```python
from build123d import *

# Parameters (mm, degrees)
SKETCH1_R                = 10
BOSS_EXTRUDE1_DEPTH      = 30
BOSS_EXTRUDE2_DEPTH      = 100
BOSS_EXTRUDE2_DEPTH_BACK = 30
SKETCH2_W                = 120
SKETCH2_H                = 25
SKETCH3_R                = 5
CUT_EXTRUDE1_DEPTH       = 70


with BuildPart() as part:
    # Sketch1 → Boss-Extrude1 (new body)
    with BuildSketch(Plane(origin=(0, 0, 0), x_dir=(0, 1, 0), z_dir=(0, 0, 1))):
        with BuildLine():
            Line((0, 60), (400, 60))
            Line((400, 60), (460, 60))
            Line((460, 60), (460, -60))
            Line((460, -60), (400, -60))
            Line((400, -60), (0, -60))
            ThreePointArc((0, -60), (-60, 0), (0, 60))
        make_face()
        with Locations(Location((0, 0, 0), (0, 0, 270))):
            Circle(SKETCH1_R, mode=Mode.SUBTRACT)
    extrude(amount=BOSS_EXTRUDE1_DEPTH)

    # Sketch2 → Boss-Extrude2 (add, two sides: drawn at the far end of the back side and taken through both)
    with BuildSketch(Plane.XY.offset(30).offset(-BOSS_EXTRUDE2_DEPTH_BACK)):
        with Locations((0, 472.5)):
            Rectangle(SKETCH2_W, SKETCH2_H)
    extrude(amount=BOSS_EXTRUDE2_DEPTH + BOSS_EXTRUDE2_DEPTH_BACK)

    # Sketch3 → Cut-Extrude1 (cut)
    with BuildSketch(Plane.XZ.offset(-460)):
        with Locations(Location((32, 77, 0), (0, 0, 270))):
            Circle(SKETCH3_R)
    extrude(amount=-CUT_EXTRUDE1_DEPTH, mode=Mode.SUBTRACT)


solid = part.part
```
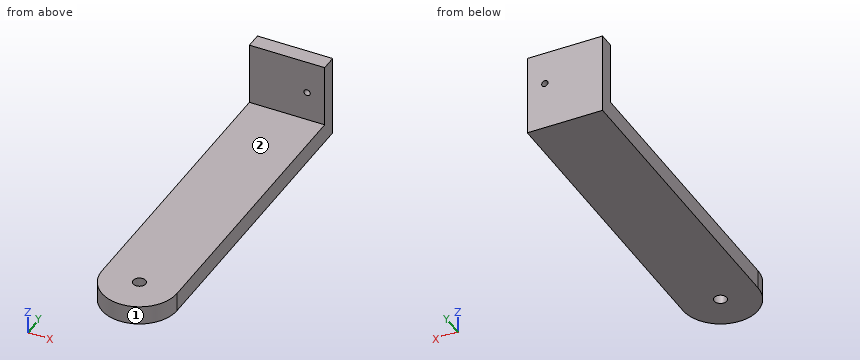
Check sheet for the modelled part. Datum: model origin and axes. Units: mm. Face numbers are marked on the shaded views. A direction names the side the tool comes from. Round coordinates to 2 decimals unless told otherwise and drop trailing zeros. Order: outer loops, then holes, each group sorted by start corner. A loop starts at its lowest first (then second) coordinate and runs counter-clockwise, first axis right, second up.
1) Tool access check on the marked faces 1 and 2. Record the directions out of +Z, -Z, +X, -X, +Y, -Y that give a thin tool (end or side, any length) a straight path to the whole face; none if there is none.
2) Section check C-C (x = 48). Record the boundary of the cut face in (y, z), and give its area (3 significant figures).
3) Section check A-A (z = 77). Record the boundary of the cut face in (x, y).
4) Go/stop test with flat-tipped pins: pin 1 Ø12 at (x, y) = (0, 0) entering from +Z; pin 2 Ø6 at (x, y) = (-13, 212) entering from +Z; pin 3 Ø12 at (x, z) = (-44.5, 53.5) entering from -Y. Record where each tip stops, or that it passes through.
5) Section check B-B (x = 0). Record the boundary of the cut face in (y, z), and give its area (4 significant figures).
6) Scan lines: line 1 (Y direction, x = 0, z = 17); line 2 (X direction, y = 477, z = 77); line 3 (Y direction, x = 25, z = 39). Record each from-to range of solid material in increasing order.
7) Section check D-D (y = 377). Record the boundary of the cut face in (x, z), and give its area (3 significant figures).
Result:
1. face 1: +Z, -Z, -Y
1. face 2: +Z, +X, -X, -Y
2. outline: (-36, 0) - (485, 0) - (485, 130) - (460, 130) - (460, 30) - (-36, 30) - close
2. area: 18,100 mm2
3. outline: (-60, 460) - (27, 460) - (27, 485) - (-60, 485) - close; (37, 460) - (60, 460) - (60, 485) - (37, 485) - close
4. pin 1: passes through
4. pin 2: stops at z = 30
4. pin 3: stops at y = 460
5. outline: (-60, 0) - (-10, 0) - (-10, 30) - (-60, 30) - close; (10, 0) - (485, 0) - (485, 130) - (460, 130) - (460, 30) - (10, 30) - close
5. area: 18,250 mm2
6. line 1: y = -60 to -10, 10 to 485
6. line 2: x = -60 to 27, 37 to 60
6. line 3: y = 460 to 485
7. outline: (-60, 0) - (60, 0) - (60, 30) - (-60, 30) - close
7. area: 3,600 mm2
